Could you check a few things on this drawing? It's one solid part, dimensions in mm from its lowest x, y, z. A direction names the side the tool comes from. Coordinates: 2 decimals unless noted, no trailing zeros. Loops run counter-clockwise (first coordinate to the right, second up) from the corner with the lowest first, then second, coordinate; pieces in that order, holes last. Notation, with made-up numbers: (19, -7.5) -> (59, -7.5) arc R9 ccw to (59, 0.5) -> close; hole circle Ø8 at (0.5, -25). An arc over 180 degrees is marked (long way). One line per question, with ' | ' between items. Start each with the question number.
(1) I'm going to push flat-ended pins straight in: pin 1 Ø4 at (x, y) = (12.5, 7) entering from -Z; pin 2 Ø3 at (y, z) = (12, 4) entering from -X; pin 3 Ø3 at (x, z) = (9, 6.5) entering from +Y; pin 4 Ø5 at (y, z) = (22.5, 5.5) entering from +X. Where does each tip first touch, or does it pass through?
(2) Suppose I cut it at C-C (z = 5). Please give me the cut outline in (x, y), plus the area to 3 significant figures.
(3) If we mould it in two halves opening along Z, with no side actions, what happens to the marked faces 4, 5 and 6? For each: pulls with the +Z half, pulls with the -Z half, needs draft (parallel to the pull), parting line crosses it, or undercut.
(4) Suppose I cut it at B-B (x = 27.25). Please give me the cut outline in (y, z).
(5) If I drill on line 1 along Z through (x, y) = (6, 1.7); line 2 along X through (y, z) = (9, 2.25); line 3 along Y through (x, z) = (27.25, 7.5), over which ranges is the centre line in solid material (lowest first)?
(6) Which directions (+Z, -Z, +X, -X, +Y, -Y) give clear straight access to the entire face, cutting with the end or side of a thin tool? Please do the marked faces 1, 2 and 3.
(7) Suppose I cut it at A-A (y = 14.25). Please give me the cut outline in (x, z), plus the area to 3 significant figures.
(8) Suppose I cut it at D-D (z = 8.75). Please give me the cut outline in (x, y).
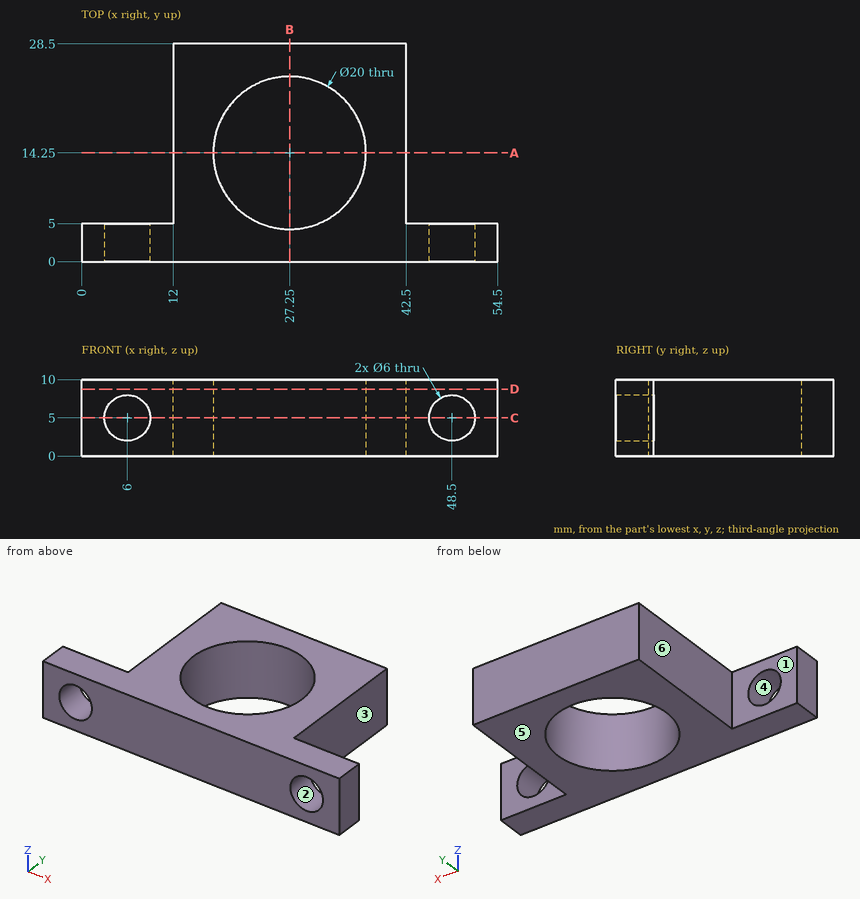
Checks:
1) pin 1: stops at z = 0 | pin 2: stops at x = 12 | pin 3: stops at y = 5 | pin 4: stops at x = 42.5
2) outline: (0, 0) -> (3, 0) -> (3, 5) -> (0, 5) -> close; (9, 0) -> (45.5, 0) -> (45.5, 5) -> (42.5, 5) -> (42.5, 28.5) -> (12, 28.5) -> (12, 5) -> (9, 5) -> close; (51.5, 0) -> (54.5, 0) -> (54.5, 5) -> (51.5, 5) -> close; hole circle Ø20 at (27.25, 14.25) | area: 615 mm^2
3) face 4: undercut | face 5: pulls with the -Z half | face 6: needs draft
4) outline: (0, 0) -> (4.25, 0) -> (4.25, 10) -> (0, 10) -> close; (24.25, 0) -> (28.5, 0) -> (28.5, 10) -> (24.25, 10) -> close
5) line 1: z = 0 to 2, 8 to 10 | line 2: x = 12 to 18.74, 35.76 to 42.5 | line 3: y = 0 to 4.25, 24.25 to 28.5
6) face 1: +Z, -Z, -X, +Y | face 2: +Y, -Y | face 3: +Z, -Z, +X, +Y
7) outline: (12, 0) -> (17.25, 0) -> (17.25, 10) -> (12, 10) -> close; (37.25, 0) -> (42.5, 0) -> (42.5, 10) -> (37.25, 10) -> close | area: 105 mm^2
8) outline: (0, 0) -> (54.5, 0) -> (54.5, 5) -> (42.5, 5) -> (42.5, 28.5) -> (12, 28.5) -> (12, 5) -> (0, 5) -> close; hole circle Ø20 at (27.25, 14.25)
